Source: CAD feature listing. Evaluate the final solid. Frame: model axes, mm. A direction names the side the tool comes from. Coordinates: 2 decimals unless noted, no trailing zeros. Write each loop counter-clockwise with the first axis right and the second up, starting at its lowest first coordinate (ties: lowest second). Pieces come first, ordered by that corner, then holes. Notation, with made-up numbers: M -14,-9.5 L 8,-9.5 A18 ccw 8,10.5 Z; hole C 38,2 d11. An arc over 180 degrees is marked long. Write item = value, one per line. Start each with the question number.
1. Section query D-D (x = 9). Output: boundary loops of the cut face in (y, z).
2. Access query for faces 5 (the face through (7, -8.1, -1)), 6 (the face through (16.4, -1, 3)), 7 (the face through (13, 0, 0)), 8 (the face through (5.3, 0, -2)), 9 (the face through (19, -5, 3)). Directions: +Z, -Z, +X, -X, +Y, -Y. A direction counts if a zero-diameter tool reaches every point of the face in a straight line with its end or side. Return the directions, or none.
3. Pull-direction query (Z, two-part tool) for faces 1 (the face through (7, 8.1, -1)), 2 (the face through (18, -1, 3.4)), 3 (the face through (6.286, 0.208, -2.414)), 4 (the face through (6, 0, -8)); classes: pulls with the +Z half, pulls with the -Z half, needs draft (parallel to the pull), parting line crosses it, or undercut.
4. Pin query (flat end, axial travel): pin 1 Ø3.5 at (y, z) = (0, -4) entering from -X; pin 2 Ø1.5 at (x, y) = (10.5, 4) entering from -Z; pin 3 Ø1.6 at (x, z) = (18, 2.5) entering from +Y; pin 4 Ø2 at (x, z) = (18, 2) entering from -Y. Return the tip coordinate at first contact, or that it passes through.
5. Section query A-A (y = 0). Output: boundary loops of the cut face in (x, z).
6. Line query: line 1 along Z through (x, y) = (6.25, 0); line 2 along Z through (x, y) = (13.25, 1); line 3 along X through (y, z) = (2.5, -3.25). Output: solid intervals per line, ascending.
7. Section query B-B (z = -4). Output: boundary loops of the cut face in (x, y), then the cut area to 3 significant figures.
8. Section query C-C (x = 7). Output: boundary loops of the cut face in (y, z), then the cut area to 3 significant figures.
```python
from build123d import *

# Parameters (mm, degrees)
F0_W      = 36
F0_H      = 16.2
F1_DEPTH  = 2.4
F2_R      = 3.5
F4_W      = 3.8
F4_H      = 2
F5_DEPTH  = 8.6
F7_W      = 14.6
F7_H      = 16.2
F8_DEPTH  = 8
F9_R      = 1.6
F10_DEPTH = 14.6
F11_START = -8.001
F6_W      = 14.9
F6_H      = 16.2
F11_DEPTH = 11.402


with BuildPart() as f1:
    # F0 (on Top) → F1 (new body)
    with BuildSketch(Plane.XY):
        Rectangle(F0_W, F0_H)
    extrude(amount=F1_DEPTH)

    # F2
    f2_edges = [f1.edges().sort_by_distance(p)[0] for p in [
        (-18, -8.1, 1.2),
        (-18, 8.1, 1.2),
        (18, -8.1, 1.2),
        (18, 8.1, 1.2),
    ]]
    fillet(f2_edges, radius=F2_R)

    # F4 (on offset) → F5 (join)
    with BuildSketch(Plane(origin=(0, 3.6, 0), x_dir=(-1, 0, 0), z_dir=(0, 1, 0))):
        with Locations((-18.3, 2.4)):
            Rectangle(F4_W, F4_H)
        with Locations((18.3, 2.4)):
            Rectangle(F4_W, F4_H)
    extrude(amount=-F5_DEPTH)

    # F7 (on face) → F8 (join)
    with BuildSketch(Plane(origin=(0, 0, 0), x_dir=(1, 0, 0), z_dir=(0, 0, -1))):
        Rectangle(F7_W, F7_H)
    extrude(amount=F8_DEPTH)

    # F9 (on face) → F10 (cut, through all)
    with BuildSketch(Plane(origin=(-7.3, 0, 0), x_dir=(0, -1, 0), z_dir=(-1, 0, 0))):
        with Locations((0, -4)):
            Circle(F9_R)
    extrude(amount=-F10_DEPTH, mode=Mode.SUBTRACT)

    # F6 (on Top) → F11 (intersect)
    with BuildSketch(Plane.XY.offset(F11_START)):
        with Locations((12.75, 0)):
            Rectangle(F6_W, F6_H)
    extrude(amount=F11_DEPTH, mode=Mode.INTERSECT)


solid = f1.part
```
Results are:
q1.outline = M -8.1,0 L 8.1,0 L 8.1,2.4 L -8.1,2.4 Z
q2.face_5 = +Z, -Z, +X, -X, -Y
q2.face_6 = +Z, -X, +Y, -Y
q2.face_7 = -Z, +X, +Y, -Y
q2.face_8 = +Z, -Z, -X, +Y, -Y
q2.face_9 = +Z, +X, -Y
q3.face_1 = needs draft
q3.face_2 = pulls with the +Z half
q3.face_3 = undercut
q3.face_4 = pulls with the -Z half
q4.pin_1 = 5.3
q4.pin_2 = 0
q4.pin_3 = 6.82
q4.pin_4 = -7.05
q5.outline = M 5.3,-8 L 7.3,-8 L 7.3,-5.6 L 5.3,-5.6 Z; M 5.3,-2.4 L 7.3,-2.4 L 7.3,0 L 18,0 L 18,1.4 L 20.2,1.4 L 20.2,3.4 L 16.4,3.4 L 16.4,2.4 L 5.3,2.4 Z
q6.line_1 = -8 to -5.6, -2.4 to 2.4
q6.line_2 = 0 to 2.4
q6.line_3 = 5.3 to 7.3
q7.outline = M 5.3,-8.1 L 7.3,-8.1 L 7.3,-1.6 L 5.3,-1.6 Z; M 5.3,1.6 L 7.3,1.6 L 7.3,8.1 L 5.3,8.1 Z
q7.area = 26.0 mm^2
q8.outline = M -8.1,-8 L 8.1,-8 L 8.1,2.4 L -8.1,2.4 Z; hole C 0,-4 d3.2
q8.area = 160 mm^2
